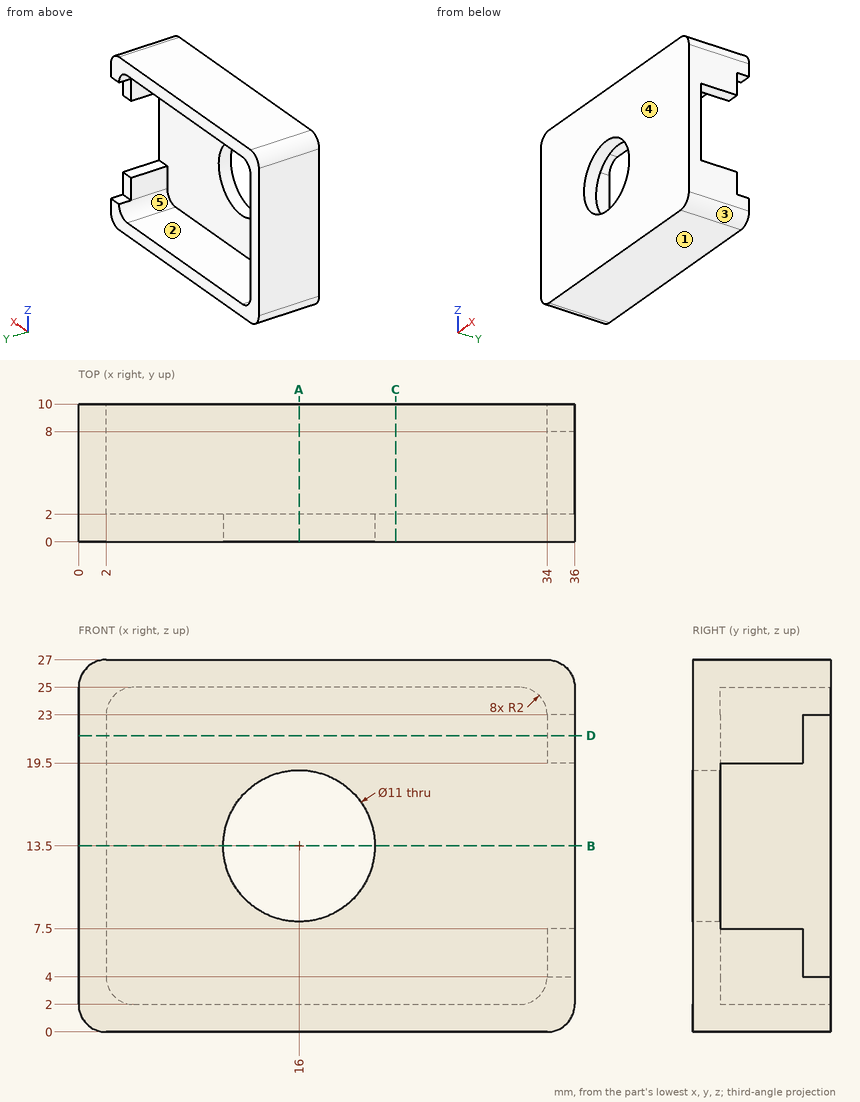
Check sheet for the drawn part. Datum: minimum x, y, z corner. Units: mm. A direction names the side the tool comes from. Round coordinates to 2 decimals unless told otherwise and drop trailing zeros. Loops run counter-clockwise (first coordinate to the right, second up) from the corner with the lowest first, then second, coordinate; pieces in that order, holes last. Notation, with made-up numbers: (11.25, -2) - (70.25, -2) arc R19 cw to (70.25, 14) - close; hole circle Ø10 at (75.5, -20). An arc over 180 degrees is marked (long way). Use one line per item in the form item = value.
1. Section check B-B on z = 13.5. Record the cut outline in (x, y).
A:
outline = (0, 0) - (10.5, 0) - (10.5, 2) - (2, 2) - (2, 10) - (0, 10) - close; (21.5, 0) - (36, 0) - (36, 2) - (21.5, 2) - close
2. Draft check along X on the marked faces 1, 2 and 3. Enter one of: pulls with the +X half, pulls with the -X half, needs draft (parallel to the pull), parting line crosses it, or undercut.
A:
face_1 = needs draft
face_2 = undercut
face_3 = pulls with the +X half
3. Access from +Z, -Z, +X, -X, +Y, -Y to the whole of each face (thin tool, end or side, straight path). Record for the marked faces 4 and 5.
A:
face_4 = +Z, -Z, +X, -X, -Y
face_5 = +Y
4. Gauge pin test, flat ends, axial feed: pin 1 Ø4 at (y, z) = (4.5, 11.5) entering from +X; pin 2 Ø1.6 at (x, y) = (35, 5.5) entering from +Z; pin 3 Ø1 at (x, y) = (35, 9) entering from +Z; pin 4 Ø9 at (x, z) = (16, 13.5) entering from -Y. Record the tip position at first contact, or that the pin passes through.
A:
pin_1 = 2
pin_2 = 26.99
pin_3 = 26.94
pin_4 = through
5. Section check A-A on x = 16. Record the cut outline in (y, z).
A:
outline = (0, 0) - (10, 0) - (10, 2) - (2, 2) - (2, 8) - (0, 8) - close; (0, 19) - (2, 19) - (2, 25) - (10, 25) - (10, 27) - (0, 27) - close
6. Section check C-C on x = 23. Record the cut outline in (y, z).
A:
outline = (0, 0) - (10, 0) - (10, 2) - (2, 2) - (2, 25) - (10, 25) - (10, 27) - (0, 27) - close
7. Scan lines: probe 1 along X at (y, z) = (0.7, 13.5); probe 2 along Z at (x, y) = (32, 6.25); probe 3 along Y at (x, z) = (7, 6). Record each from-to range of solid material in increasing order.
A:
probe_1 = 0 to 10.5, 21.5 to 36
probe_2 = 0 to 2, 25 to 27
probe_3 = 0 to 2
8. Section check D-D on z = 21.5. Record the cut outline in (x, y).
A:
outline = (0, 0) - (36, 0) - (36, 8) - (34, 8) - (34, 2) - (2, 2) - (2, 10) - (0, 10) - close
